from build123d import *

# Parameters (mm, degrees)
F1_DEPTH = 3
F2_R     = 39.5
F3_DEPTH = 40
F4_R     = 1.5
F5_DEPTH = 3
F5_TAPER = 5
F6_R     = 1
F7_R     = 37.5
F8_DEPTH = 40


with BuildPart() as f1:
    # F0 (on Front) → F1 (new body)
    with BuildSketch(Plane.XZ):
        with BuildLine():
            Line((0, 21), (0, 0))
            Line((0, 0), (7, 0))
            ThreePointArc((7, 0), (7.7639320225, 8.472135955), (15, 4))
            ThreePointArc((15, 4), (14.472135955, 1.7639320225), (13, 0))
            Line((13, 0), (51, 0))
            ThreePointArc((51, 0), (49.2565835097, 5.5811388301), (54, 9))
            Line((54, 9), (54, 44))
            Line((54, 44), (0, 44))
            Line((0, 44), (0, 27))
            ThreePointArc((0, 27), (5.5811388301, 28.7434164903), (9, 24))
            ThreePointArc((9, 24), (5.5811388301, 19.2565835097), (0, 21))
        make_face()
        with BuildLine():
            ThreePointArc((15, 4), (7.7639320225, 8.472135955), (7, 0))
            Line((7, 0), (13, 0))
            ThreePointArc((13, 0), (14.472135955, 1.7639320225), (15, 4))
        make_face()
        with BuildLine():
            Line((13, 0), (7, 0))
            ThreePointArc((7, 0), (10, -1), (13, 0))
        make_face()
        with BuildLine():
            ThreePointArc((0, 27), (-1, 24), (0, 21))
            Line((0, 21), (0, 27))
        make_face()
        with BuildLine():
            Line((0, 27), (0, 21))
            ThreePointArc((0, 21), (5.5811388301, 19.2565835097), (9, 24))
            ThreePointArc((9, 24), (5.5811388301, 28.7434164903), (0, 27))
        make_face()
        with BuildLine():
            ThreePointArc((54, 9), (49.2565835097, 5.5811388301), (51, 0))
            Line((51, 0), (54, 0))
            Line((54, 0), (54, 9))
        make_face()
        with BuildLine():
            Line((54, 0), (51, 0))
            ThreePointArc((51, 0), (54, -1), (57, 0))
            Line((57, 0), (54, 0))
        make_face()
        with BuildLine():
            Line((0, 61), (0, 44))
            Line((0, 44), (54, 44))
            Line((54, 44), (54, 79))
            ThreePointArc((54, 79), (49.2565835097, 82.4188611699), (51, 88))
            Line((51, 88), (13, 88))
            ThreePointArc((13, 88), (14.472135955, 86.2360679775), (15, 84))
            ThreePointArc((15, 84), (7.7639320225, 79.527864045), (7, 88))
            Line((7, 88), (0, 88))
            Line((0, 88), (0, 67))
            ThreePointArc((0, 67), (5.5811388301, 68.7434164903), (9, 64))
            ThreePointArc((9, 64), (5.5811388301, 59.2565835097), (0, 61))
        make_face()
        with BuildLine():
            Line((54, 9), (54, 0))
            Line((54, 0), (57, 0))
            ThreePointArc((57, 0), (58.472135955, 1.7639320225), (59, 4))
            ThreePointArc((59, 4), (57.5355339059, 7.5355339059), (54, 9))
        make_face()
        with BuildLine():
            Line((54, 44), (54, 9))
            ThreePointArc((54, 9), (57.5355339059, 7.5355339059), (59, 4))
            ThreePointArc((59, 4), (58.472135955, 1.7639320225), (57, 0))
            Line((57, 0), (95, 0))
            ThreePointArc((95, 0), (95.7639320225, 8.472135955), (103, 4))
            ThreePointArc((103, 4), (102.472135955, 1.7639320225), (101, 0))
            Line((101, 0), (108, 0))
            Line((108, 0), (108, 21))
            ThreePointArc((108, 21), (99, 24), (108, 27))
            Line((108, 27), (108, 44))
            Line((108, 44), (54, 44))
        make_face()
        with BuildLine():
            ThreePointArc((0, 67), (-1, 64), (0, 61))
            Line((0, 61), (0, 67))
        make_face()
        with BuildLine():
            Line((0, 67), (0, 61))
            ThreePointArc((0, 61), (5.5811388301, 59.2565835097), (9, 64))
            ThreePointArc((9, 64), (5.5811388301, 68.7434164903), (0, 67))
        make_face()
        with BuildLine():
            Line((54, 79), (54, 44))
            Line((54, 44), (108, 44))
            Line((108, 44), (108, 61))
            ThreePointArc((108, 61), (99, 64), (108, 67))
            Line((108, 67), (108, 88))
            Line((108, 88), (101, 88))
            ThreePointArc((101, 88), (102.472135955, 86.2360679775), (103, 84))
            ThreePointArc((103, 84), (95.7639320225, 79.527864045), (95, 88))
            Line((95, 88), (57, 88))
            ThreePointArc((57, 88), (58.472135955, 86.2360679775), (59, 84))
            ThreePointArc((59, 84), (57.5355339059, 80.4644660941), (54, 79))
        make_face()
        with BuildLine():
            ThreePointArc((103, 4), (95.7639320225, 8.472135955), (95, 0))
            Line((95, 0), (101, 0))
            ThreePointArc((101, 0), (102.472135955, 1.7639320225), (103, 4))
        make_face()
        with BuildLine():
            Line((101, 0), (95, 0))
            ThreePointArc((95, 0), (98, -1), (101, 0))
        make_face()
        with BuildLine():
            ThreePointArc((51, 88), (49.2565835097, 82.4188611699), (54, 79))
            Line((54, 79), (54, 88))
            Line((54, 88), (51, 88))
        make_face()
        with BuildLine():
            Line((54, 88), (54, 79))
            ThreePointArc((54, 79), (57.5355339059, 80.4644660941), (59, 84))
            ThreePointArc((59, 84), (58.472135955, 86.2360679775), (57, 88))
            Line((57, 88), (54, 88))
        make_face()
        with BuildLine():
            Line((51, 88), (54, 88))
            Line((54, 88), (57, 88))
            ThreePointArc((57, 88), (54, 89), (51, 88))
        make_face()
        with BuildLine():
            ThreePointArc((109, 24), (108.7434164903, 25.5811388301), (108, 27))
            Line((108, 27), (108, 21))
            ThreePointArc((108, 21), (108.7434164903, 22.4188611699), (109, 24))
        make_face()
        with BuildLine():
            Line((108, 21), (108, 27))
            ThreePointArc((108, 27), (99, 24), (108, 21))
        make_face()
        with BuildLine():
            ThreePointArc((108, 67), (99, 64), (108, 61))
            Line((108, 61), (108, 67))
        make_face()
        with BuildLine():
            Line((108, 67), (108, 61))
            ThreePointArc((108, 61), (108.7434164903, 62.4188611699), (109, 64))
            ThreePointArc((109, 64), (108.7434164903, 65.5811388301), (108, 67))
        make_face()
        with BuildLine():
            ThreePointArc((13, 88), (10, 89), (7, 88))
            Line((7, 88), (13, 88))
        make_face()
        with BuildLine():
            Line((13, 88), (7, 88))
            ThreePointArc((7, 88), (7.7639320225, 79.527864045), (15, 84))
            ThreePointArc((15, 84), (14.472135955, 86.2360679775), (13, 88))
        make_face()
        with BuildLine():
            ThreePointArc((101, 88), (98, 89), (95, 88))
            Line((95, 88), (101, 88))
        make_face()
        with BuildLine():
            Line((101, 88), (95, 88))
            ThreePointArc((95, 88), (95.7639320225, 79.527864045), (103, 84))
            ThreePointArc((103, 84), (102.472135955, 86.2360679775), (101, 88))
        make_face()
    extrude(amount=F1_DEPTH)

    # F2 (on face) → F3 (join)
    with BuildSketch(Plane(origin=(0, 0, 0), x_dir=(-1, 0, 0), z_dir=(0, 1, 0))):
        with Locations((-54, 44)):
            Circle(F2_R)
    extrude(amount=F3_DEPTH)

    # F4 (on face) → F5 (join)
    with BuildSketch(Plane(origin=(0, 0, 0), x_dir=(-1, 0, 0), z_dir=(0, 1, 0))):
        with Locations((-85.5000000012, 77)):
            Circle(F4_R)
        with Locations((-22.4999999988, 77)):
            Circle(F4_R)
        with Locations((-85.5000000012, 11)):
            Circle(F4_R)
        with Locations((-22.4999999988, 11)):
            Circle(F4_R)
    extrude(amount=F5_DEPTH, taper=F5_TAPER)

    # F6
    f6_edges = [f1.edges().sort_by_distance(p)[0] for p in [
        (93.5, 40, 44),
    ]]
    fillet(f6_edges, radius=F6_R)

    # F7 (on face) → F8 (cut)
    with BuildSketch(Plane.XZ.offset(3)):
        with Locations((54, 44)):
            Circle(F7_R)
    extrude(amount=-F8_DEPTH, mode=Mode.SUBTRACT)


solid = f1.part
Design review of the part built by this model. Coordinates are the model's own, in mm. A direction names the side the tool comes from. Coordinates: 2 decimals unless noted, no trailing zeros. Write each loop counter-clockwise with the first axis right and the second up, starting at its lowest first coordinate (ties: lowest second). Pieces come first, ordered by that corner, then holes. Notation, with made-up numbers: (36, 69.5) - (91, 69.5) arc R25 ccw to (91, 85.5) - close; hole circle Ø10 at (18.5, 12.5). An arc over 180 degrees is marked (long way). Use one line per item in the form item = value.
Q1. Consider section C-C (y = 17.5). Write out the cut boundary in (x, z), plus the area to 3 significant figures.
Taken from the geometry:
outline = circle Ø79 at (54, 44); hole circle Ø75 at (54, 44)
area = 484 mm^2
Q2. For probe 1 along Y at (x, z) = (41.5, 78); probe 2 along Y at (x, z) = (34, 80); probe 3 along Z at (x, y) = (54, 12), list the stretches that pass through material, from the lowest coordinate up.
Taken from the geometry:
probe_1 = 37 to 40
probe_2 = -3 to 0
probe_3 = 4.5 to 6.5, 81.5 to 83.5
Q3. The part is to be moulded in two halves that separate along Z. For faces 4 (the flat face through (108, -1, 10)), 5 (the flat face through (53, 37, 45)), 6 (the cylindrical face through (10, -1, 89)), say which applies: +Z half, -Z half, draft (parallel to the pull), parting line (faces both ways), or undercut.
Taken from the geometry:
face_4 = draft
face_5 = undercut
face_6 = +Z half
Q4. Consider section A-A (z = 44). Write out the cut boundary in (x, y).
Taken from the geometry:
outline = (0, -3) - (16.5, -3) - (16.5, 37) - (91.5, 37) - (91.5, -3) - (108, -3) - (108, 0) - (93.5, 0) - (93.5, 39) arc R1 ccw to (92.5, 40) - (15.5, 40) arc R1 ccw to (14.5, 39) - (14.5, 0) - (0, 0) - close
Q5. Consider section B-B (x = 54). Write out the cut boundary in (y, z).
Taken from the geometry:
outline = (-3, -1) - (0, -1) - (0, 4.5) - (39, 4.5) arc R1 ccw to (40, 5.5) - (40, 82.5) arc R1 ccw to (39, 83.5) - (0, 83.5) - (0, 89) - (-3, 89) - (-3, 81.5) - (37, 81.5) - (37, 6.5) - (-3, 6.5) - close
Q6. Insertion check: pin 1 Ø6 at (y, z) = (25.5, 37) entering from -X; pin 2 Ø8 at (x, y) = (90.5, 27.5) entering from -Z; pin 3 Ø1 at (x, z) = (88, 30) entering from -Y. Each pin has a flat end and moves straight along its axis. Give the tip position at first contact, or say it passes through.
Taken from the geometry:
pin_1 = 14.7
pin_2 = 21.55
pin_3 = 37
Q7. Machinability: for faces 1 (the flat face through (4, -1, 88)), 2 (the flat face through (86, 3, 77)), 3 (the flat face through (108, -1, 77)), which of the approach directions +Z, -Z, +X, -X, +Y, -Y give a long, thin tool a straight path to every point of the face, cutting with its end or side? Answer none if there is none.
Taken from the geometry:
face_1 = +Z, -X, +Y, -Y
face_2 = +Z, +X, +Y
face_3 = +Z, +X, +Y, -Y
